from build123d import *

# Parameters (mm, degrees)
SKETCH_1_W          = 186
SKETCH_1_H          = 20
EXTRUDE_1_DEPTH     = 15
EXTRUDE_1_DRAFT     = -18
SKETCH_2_W          = 186
SKETCH_2_H          = 20
CUT_EXTRUDE_2_DEPTH = 2
SKETCH_3_W          = 177
SKETCH_3_H          = 13
CUT_EXTRUDE_3_DEPTH = 4
SKETCH_4_R          = 2.75
CUT_EXTRUDE_6_DEPTH = 5.5


with BuildPart() as part:
    # 草图1 → 凸台-拉伸1 (with draft: the straight prism first)
    with BuildSketch(Plane(origin=(0, 0, 0), x_dir=(1, 0, 0), z_dir=(0, 1, 0))):
        Rectangle(SKETCH_1_W, SKETCH_1_H)
    extrude(amount=EXTRUDE_1_DEPTH)
    # 凸台-拉伸1: the draft: its side faces are tilted about the plane it starts from
    extrude_1_sides = [part.faces().sort_by_distance(p)[0] for p in [
        (-93, 7.5, 0),
        (0, 7.5, 10),
        (93, 7.5, 0),
        (0, 7.5, -10),
    ]]
    draft(extrude_1_sides, Plane(origin=(0, 0, 0), x_dir=(1, 0, 0), z_dir=(0, 1, 0)), EXTRUDE_1_DRAFT)

    # 草图2 → 切除-拉伸2 (cut)
    with BuildSketch(Plane(origin=(0, 15, 0), x_dir=(1, 0, 0), z_dir=(0, 1, 0))):
        Rectangle(SKETCH_2_W, SKETCH_2_H)
    extrude(amount=-CUT_EXTRUDE_2_DEPTH, mode=Mode.SUBTRACT)

    # 草图3 → 切除-拉伸3 (cut)
    with BuildSketch(Plane.XZ):
        Rectangle(SKETCH_3_W, SKETCH_3_H)
    extrude(amount=-CUT_EXTRUDE_3_DEPTH, mode=Mode.SUBTRACT)

    # 草图4 → 切除-拉伸6 (cut)
    with BuildSketch(Plane.XZ.offset(-4)):
        with Locations(Location((-72, 0, 0), (0, 0, 270))):
            Circle(SKETCH_4_R)
        with Locations(Location((-38, 0, 0), (0, 0, 270))):
            Circle(SKETCH_4_R)
        with Locations(Location((38, 0, 0), (0, 0, 270))):
            Circle(SKETCH_4_R)
        with Locations(Location((72, 0, 0), (0, 0, 270))):
            Circle(SKETCH_4_R)
    extrude(amount=-CUT_EXTRUDE_6_DEPTH, mode=Mode.SUBTRACT)


solid = part.part
Here's how the part is built. I have some questions about the finished solid (model axes, mm). A direction names the side the tool comes from. Give positions to 0.01 mm unless a question says otherwise; leave off trailing zeros. Order: outer loops, then holes, each group sorted by start corner. A loop starts at its lowest first (then second) coordinate and runs counter-clockwise, first axis right, second up. Notation, with made-up numbers: (41, 85.5) -> (75, 85.5) arc R21 cw to (75, 109.5) -> close; hole circle Ø4 at (44.25, 35.5). An arc over 180 degrees is marked (long way). One line per item, written item: value. Start each with the question number.
1. Imagine slicing it at C-C, the plane y = 7.25. List the corners of the cut face in (x, z) for me, plus the area to 3 significant figures.
2. Imagine slicing it at A-A, the plane z = 0. List the corners of the cut face in (x, y) for me.
3. We'd pull the mould along X, two halves only. Please class faces 1 (the face through (-95.403, 7.395, 0.208)), 2 (the face through (95.403, 7.395, 0.208)), 3 (the face through (-1, 2, 6.5)): released by +X, released by -X, zero draft, split by the parting line, or undercut.
4. I need wall thicknesses on probe 1 along X at (y, z) = (7.85, 0); probe 2 along X at (y, z) = (6.25, 0); probe 3 along Y at (x, z) = (28, -2.25). Which ranges of each line are inside material? Lowest first, please. Write a range as from..to.
5. Will these pins go through, and if not, where does the flat tip stop? pin 1 Ø1 at (x, y) = (76, 10.5) entering from -Z; pin 2 Ø1.2 at (x, y) = (34, 2) entering from +Z; pin 3 Ø3 at (x, z) = (38, 0) entering from -Y.
6. Imagine slicing it at B-B, the plane x = 38. List the corners of the cut face in (y, z) for me.
7. For faces 4 (the face through (-1, 0, -7)), 5 (the face through (-1, 13, 0)), 6 (the face through (-72, 9.5, 0)), which set-ups out of +Z, -Z, +X, -X, +Y, -Y let a thin tool reach every point of the face, with its end or its side?
8. Imagine slicing it at D-D, the plane x = -28.5. List the corners of the cut face in (y, z) for me, plus the area to 3 significant figures.
Values follow:
1. outline: (-95.36, -12.36) -> (95.36, -12.36) -> (95.36, 12.36) -> (-95.36, 12.36) -> close; hole circle Ø5.5 at (-72, 0); hole circle Ø5.5 at (-38, 0); hole circle Ø5.5 at (38, 0); hole circle Ø5.5 at (72, 0)
1. area: 4,620 mm2
2. outline: (-97.87, 15) -> (-93, 0) -> (-88.5, 0) -> (-88.5, 4) -> (-74.75, 4) -> (-74.75, 9.5) -> (-69.25, 9.5) -> (-69.25, 4) -> (-40.75, 4) -> (-40.75, 9.5) -> (-35.25, 9.5) -> (-35.25, 4) -> (35.25, 4) -> (35.25, 9.5) -> (40.75, 9.5) -> (40.75, 4) -> (69.25, 4) -> (69.25, 9.5) -> (74.75, 9.5) -> (74.75, 4) -> (88.5, 4) -> (88.5, 0) -> (93, 0) -> (97.87, 15) -> (93, 15) -> (93, 13) -> (-93, 13) -> (-93, 15) -> close
3. face 1: released by -X
3. face 2: released by +X
3. face 3: undercut
4. probe 1: x = -95.55..-74.75, -69.25..-40.75, -35.25..35.25, 40.75..69.25, 74.75..95.55
4. probe 2: x = -95.03..-74.75, -69.25..-40.75, -35.25..35.25, 40.75..69.25, 74.75..95.03
4. probe 3: y = 4..13
5. pin 1: stops at z = -13.57
5. pin 2: stops at z = 10.84
5. pin 3: stops at y = 9.5
6. outline: (0, -10) -> (15, -14.87) -> (15, -10) -> (13, -10) -> (13, 10) -> (15, 10) -> (15, 14.87) -> (0, 10) -> (0, 6.5) -> (4, 6.5) -> (4, 2.75) -> (9.5, 2.75) -> (9.5, -2.75) -> (4, -2.75) -> (4, -6.5) -> (0, -6.5) -> close
7. face 4: +Z, -Z, +X, -X, -Y
7. face 5: +Y
7. face 6: -Y
8. outline: (0, -10) -> (15, -14.87) -> (15, -10) -> (13, -10) -> (13, 10) -> (15, 10) -> (15, 14.87) -> (0, 10) -> (0, 6.5) -> (4, 6.5) -> (4, -6.5) -> (0, -6.5) -> close
8. area: 281 mm2
